```python
from build123d import *

# Parameters (mm, degrees)
EXTRUDE015_DEPTH = 27.5
EXTRUDE_DEPTH    = 17


with BuildPart() as extrude015:
    # Sketch020 → Extrude015 (new body)
    with BuildSketch(Plane(origin=(-6, 0, 0), x_dir=(0, -1, 0), z_dir=(-1, 0, 0))):
        Polygon((19.5, -10.1), (19.5, -9.1), (5, -9.1), (4, -10.1), align=None)
    extrude(amount=EXTRUDE015_DEPTH)


with BuildPart() as cut006:
    # Sketch001 → Extrude (new body)
    with BuildSketch(Plane.XZ.offset(25)):
        with BuildLine():
            ThreePointArc((-8.6, 0), (-6.081118, -6.081118), (0, -8.6))
            Line((0, -8.6), (0, -9.6))
            Line((0, -9.6), (-34.5, -9.6))
            Line((-34.5, -9.6), (-34.5, -5.6))
            Line((-33.5, -5.6), (-34.5, -5.6))
            Line((-33.5, -6.6), (-33.5, -5.6))
            Line((-33.5, -6.6), (-9.5, -6.6))
            ThreePointArc((-9.5, -6.6), (-8.25, -5.35), (-9.5, -4.1))
            Line((-9.5, -4.1), (-20.83, -4.1))
            Line((-20.83, -4.1), (-20.83, -2.1))
            Line((-20.83, -2.1), (-11.7, -2.1))
            ThreePointArc((-11.7, -2.1), (-10.215076, -1.484924), (-9.6, 0))
            Line((-9.6, 0), (-8.6, 0))
        make_face()
    extrude(amount=-EXTRUDE_DEPTH)


with BuildPart() as cut006_1:
    # Extrude placement: moved
    add(cut006.part.moved(Location((0, 4.5, 0))))

    # Cut006: cut Extrude015
    add(extrude015.part, mode=Mode.SUBTRACT)


solid = cut006_1.part
```
Work out the finished part from the listing and answer in its coordinate system (mm). A direction names the side the tool comes from. Give positions to 0.01 mm unless a question says otherwise; leave off trailing zeros. Loops run counter-clockwise (first coordinate to the right, second up) from the corner with the lowest first, then second, coordinate; pieces in that order, holes last. Notation, with made-up numbers: M 62.5,-15.75 L 77.5,-15.75 A8 ccw 77.5,-7.75 Z; hole C 88,-29.5 d8. An arc over 180 degrees is marked long. One line per item, written item: value. Start each with the question number.
1. Which of the six approach directions +Z, -Z, +X, -X, +Y, -Y give full straight-line access (tool end or side, diameter ignored) to faces 1 (the face through (-34, -12, -5.6)), 2 (the face through (-33.5, -12, -6)), 3 (the face through (-15, -12, -4.1)), 4 (the face through (-8.25, -12.12, -5.38))?
2. Each of these flat-tipped pins is pushed along its axis until it touches: P1, Ø1.1, axis at x = -34, y = -12, coming from the +Z side; P2, Ø6, axis at x = -21.5, y = -18, coming from the -Z side; P3, Ø4, axis at x = -15.5, y = -8.5, coming from the +Z side; P4, Ø7.5, axis at x = -14.5, y = -15.5, coming from the +Z side. Where does it stop, or does it pass through?
3. Find section D-D (x = -11). Give the vertices of the cut face in (y, z).
4. Find the intervals of material crossed by probe 1 along Z at (x, y) = (-13, -14.75); probe 2 along Z at (x, y) = (-9.5, -5.25); probe 3 along Z at (x, y) = (-29, -18.5), in increasing order.
5. Find section A-A (x = -15.5). Give the vertices of the cut face in (y, z).
6. Find section B-B (y = -7). Give the vertices of the cut face in (x, z), and give its area (3 significant figures).
7. Find section C-C (x = -22.5). Give the vertices of the cut face in (y, z).
8. Determine the mould class of faces 5 (the face through (-16, -12, -2.1)), 6 (the face through (0, -12, -9)), 7 (the face through (-22, -12, -6.6)) for opening direction Z: released by +Z, released by -Z, zero draft, split by the parting line, or undercut.
Reported:
1. face 1: +Z, -X, +Y, -Y
1. face 2: +Z, +Y, -Y
1. face 3: -X, +Y, -Y
1. face 4: +Y, -Y
2. P1: stops at z = -5.6
2. P2: stops at z = -9.6
2. P3: stops at z = -2.1
2. P4: stops at z = -1.87
3. outline: M -20.5,-9.6 L -19.5,-9.6 L -19.5,-9.1 L -5,-9.1 L -4.5,-9.6 L -3.5,-9.6 L -3.5,-6.6 L -20.5,-6.6 Z; M -20.5,-4.1 L -3.5,-4.1 L -3.5,-1.98 L -20.5,-1.98 Z
4. probe 1: z = -9.1 to -6.6, -4.1 to -2.1
4. probe 2: z = -9.1 to -6.6, -4.1 to 0
4. probe 3: z = -9.1 to -6.6
5. outline: M -20.5,-9.6 L -19.5,-9.6 L -19.5,-9.1 L -5,-9.1 L -4.5,-9.6 L -3.5,-9.6 L -3.5,-6.6 L -20.5,-6.6 Z; M -20.5,-4.1 L -3.5,-4.1 L -3.5,-2.1 L -20.5,-2.1 Z
6. outline: M -34.5,-9.6 L -33.5,-9.6 L -33.5,-9.1 L -6,-9.1 L -6,-9.6 L 0,-9.6 L 0,-8.6 A8.6 cw -8.6,0 L -9.6,0 A2.1 cw -11.7,-2.1 L -20.83,-2.1 L -20.83,-4.1 L -9.5,-4.1 A1.25 cw -9.5,-6.6 L -33.5,-6.6 L -33.5,-5.6 L -34.5,-5.6 Z
6. area: 117 mm²
7. outline: M -20.5,-9.6 L -19.5,-9.6 L -19.5,-9.1 L -5,-9.1 L -4.5,-9.6 L -3.5,-9.6 L -3.5,-6.6 L -20.5,-6.6 Z
8. face 5: released by +Z
8. face 6: zero draft
8. face 7: undercut
